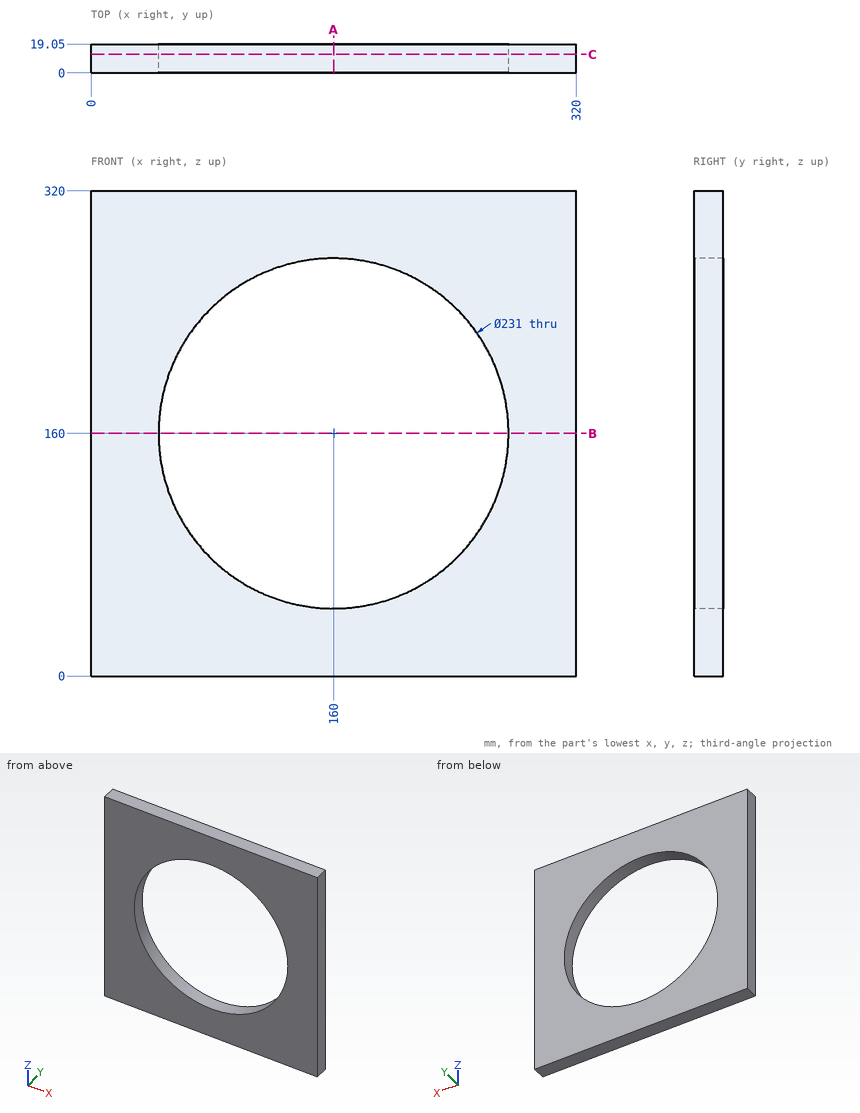
Here's the drawing with two shaded views (mm, measured from the low corner). I have some questions. Give positions to 0.01 mm unless a question says otherwise; leave off trailing zeros. Write each loop counter-clockwise with the first axis right and the second up, starting at its lowest first coordinate (ties: lowest second). Pieces come first, ordered by that corner, then holes. Notation, with made-up numbers: (39, 32.25) -> (96, 32.25) arc R14 ccw to (96, 40.25) -> close; hole circle Ø6 at (51, -1.5). An arc over 180 degrees is marked (long way). Answer as a JSON object with one key per item and string values. Group by question number.
Item 1: Suppose I cut it at A-A (x = 160). Please give me the cut outline in (y, z).
Item 2: Please list where these lines run through material, in increasing order: line 1 (X direction, y = 1.75, z = 164); line 2 (Z direction, x = 160, y = 10.25); line 3 (X direction, y = 7, z = 241.5). Write a range as [from, to].
Item 3: Suppose I cut it at C-C (y = 12.25). Please give me the cut outline in (x, z).
Item 4: Suppose I cut it at B-B (z = 160). Please give me the cut outline in (x, y), plus the area to 3 significant figures.
Findings:
{
 "1": {"outline": "(0, 0) -> (19.05, 0) -> (19.05, 44.5) -> (0, 44.5) -> close; (0, 275.5) -> (19.05, 275.5) -> (19.05, 320) -> (0, 320) -> close"},
 "2": {"line 1": "x = [0, 44.57], [275.43, 320]", "line 2": "z = [0, 44.5], [275.5, 320]", "line 3": "x = [0, 78.16], [241.84, 320]"},
 "3": {"outline": "(0, 0) -> (320, 0) -> (320, 320) -> (0, 320) -> close; hole circle Ø231 at (160, 160)"},
 "4": {"outline": "(0, 0) -> (44.5, 0) -> (44.5, 19.05) -> (0, 19.05) -> close; (275.5, 0) -> (320, 0) -> (320, 19.05) -> (275.5, 19.05) -> close", "area": "1,700 mm²"}
}
